```python
from build123d import *

# Parameters (mm, degrees)
BOSS_EXTRUDE1_DEPTH = 2.5
FILLET1_R           = 3


with BuildPart() as part:
    # Sketch1 → Boss-Extrude1 (new body, symmetric)
    with BuildSketch(Plane.XY):
        with BuildLine():
            Line((-7.5, 213), (-17.5, 213))
            Line((-17.5, 213), (-17.5, 197))
            ThreePointArc((-17.5, 197), (-25, 189.5), (-32.5, 197))
            Line((-32.5, 197), (-32.5, 213))
            Line((-32.5, 213), (-50, 213))
            Line((-50, 213), (-50, 0))
            Line((-50, 0), (50, 0))
            Line((50, 0), (50, 213))
            Line((50, 213), (32.5, 213))
            Line((32.5, 213), (32.5, 197))
            ThreePointArc((32.5, 197), (25, 189.5), (17.5, 197))
            Line((17.5, 197), (17.5, 213))
            Line((17.5, 213), (7.5, 213))
            Line((7.5, 213), (7.5, 197))
            ThreePointArc((7.5, 197), (0, 189.5), (-7.5, 197))
            Line((-7.5, 197), (-7.5, 213))
        make_face()
    extrude(amount=BOSS_EXTRUDE1_DEPTH, both=True)

    # Fillet1
    fillet1_edges = [part.edges().sort_by_distance(p)[0] for p in [
        (50, 213, 0),
        (50, 0, 0),
        (-50, 0, 0),
        (-50, 213, 0),
    ]]
    fillet(fillet1_edges, radius=FILLET1_R)


solid = part.part
```
Check sheet for the modelled part. Datum: model origin and axes. Units: mm. A direction names the side the tool comes from. Round coordinates to 2 decimals unless told otherwise and drop trailing zeros. Write each loop counter-clockwise with the first axis right and the second up, starting at its lowest first coordinate (ties: lowest second). Pieces come first, ordered by that corner, then holes. Notation, with made-up numbers: M -21.5,-28 L 31.5,-28 A31 ccw 31.5,11 Z; hole C -13,29.25 d8. An arc over 180 degrees is marked long. Write item = value, one per line. Start each with the question number.
1. Tool access check on faces 1 (the flat face through (-17.5, 205, 0)), 2 (the flat face through (50, 105, 0)). Record the directions out of +Z, -Z, +X, -X, +Y, -Y that give a thin tool (end or side, any length) a straight path to the whole face; none if there is none.
2. Release check for a two-part mould opening along X. For faces 3 (the flat face through (32.5, 205, 0)), 4 (the cylindrical face through (25.16, 189.5, 0.04)), 5 (the flat face through (-12, 213, 0)), 6 (the flat face through (-50, 108, 0)) record: pulls with the +X half, pulls with the -X half, needs draft (parallel to the pull), parting line crosses it, or undercut.
3. Section check A-A, the plane z = -0.5. Record the cut outline in (x, y).
4. Scan lines: line 1 (X direction, y = 195.5, z = -1.5); line 2 (Y direction, x = 23.5, z = 0.65); line 3 (Y direction, x = 18.5, z = 0.85). Record each from-to range of solid material in increasing order. Write a range as [from, to].
5. Section check C-C, the plane x = 25. Record the cut outline in (y, z).
6. Section check B-B, the plane x = -21.5. Record the cut outline in (y, z).
Results found:
q1.face_1 = +Z, -Z, +Y
q1.face_2 = +Z, -Z, +X, +Y, -Y
q2.face_3 = undercut
q2.face_4 = undercut
q2.face_5 = needs draft
q2.face_6 = pulls with the -X half
q3.outline = M -50,3 A3 ccw -47,0 L 47,0 A3 ccw 50,3 L 50,210 A3 ccw 47,213 L 32.5,213 L 32.5,197 A7.5 cw 17.5,197 L 17.5,213 L 7.5,213 L 7.5,197 A7.5 cw -7.5,197 L -7.5,213 L -17.5,213 L -17.5,197 A7.5 cw -32.5,197 L -32.5,213 L -47,213 A3 ccw -50,210 Z
q4.line_1 = [-50, -32.35], [-17.65, -7.35], [7.35, 17.65], [32.35, 50]
q4.line_2 = [0, 189.65]
q4.line_3 = [0, 193.26]
q5.outline = M 0,-2.5 L 189.5,-2.5 L 189.5,2.5 L 0,2.5 Z
q6.outline = M 0,-2.5 L 190.37,-2.5 L 190.37,2.5 L 0,2.5 Z
